Check sheet for the modelled part. Datum: model origin and axes. Units: mm. Face numbers are marked on the shaded views. A direction names the side the tool comes from. Round coordinates to 2 decimals unless told otherwise and drop trailing zeros. Order: outer loops, then holes, each group sorted by start corner. A loop starts at its lowest first (then second) coordinate and runs counter-clockwise, first axis right, second up. Notation, with made-up numbers: (-20, 56.5) -> (37, 56.5) arc R16 cw to (37, 60.5) -> close; hole circle Ø8 at (38, -35.5). An arc over 180 degrees is marked (long way). Answer in a Markdown table with one row per item. Add a question column.
1. Access from +Z, -Z, +X, -X, +Y, -Y to the whole of each face (thin tool, end or side, straight path). Record for the marked faces 1 and 2.
2. Material ranges on L1, parallel to Z at x = -0.5, y = 2.25; L2, parallel to Z at x = 1.25, y = 0; L3, parallel to X at y = 1.25, z = 11, recorded low to high. Write a range as from..to.
3. Depth check by flat-ended pin: P1, Ø1, axis at x = -2, y = -1, coming from the -Z side; P2, Ø1, axis at x = -1.5, z = 5, coming from the -Y side. Enter the tip coordinate at first touch or a pass-through.
4. Sectioned sample at D-D, the plane z = 9.75. Record the boundary of the cut face in (x, y), then the cut area to 3 significant figures.
5. Draft check along Y on the marked faces 3, 4 and 5. Enter one of: +Y half, -Y half, draft (parallel to the pull), parting line (faces both ways), or undercut.
6. Sectioned sample at C-C, the plane z = 1.5. Record the boundary of the cut face in (x, y).
7. Sectioned sample at A-A, the plane y = 0. Record the boundary of the cut face in (x, z).
8. Sectioned sample at B-B, the plane x = 1.25. Record the boundary of the cut face in (y, z).
```python
from build123d import *

# Parameters (mm, degrees)
SKETCH_1_R          = 1.5
EXTRUDE_1_DEPTH     = 6
SKETCH_2_R          = 2
EXTRUDE_2_DEPTH     = 8
SKETCH_3_R          = 3.5
EXTRUDE_3_DEPTH     = 3.5
CUT_EXTRUDE_1_DEPTH = 2


with BuildPart() as part:
    # 草图1 → 凸台-拉伸1 (new body)
    with BuildSketch(Plane.XY):
        Circle(SKETCH_1_R)
    extrude(amount=EXTRUDE_1_DEPTH)

    # 草图2 → 凸台-拉伸2 (add)
    with BuildSketch(Plane.XY.offset(6)):
        Circle(SKETCH_2_R)
    extrude(amount=EXTRUDE_2_DEPTH)

    # 草图3 → 凸台-拉伸3 (add)
    with BuildSketch(Plane.XY.offset(14)):
        Circle(SKETCH_3_R)
    extrude(amount=EXTRUDE_3_DEPTH)

    # 草图4 → 切除-拉伸1 (cut)
    with BuildSketch(Plane.XY.offset(17.5)):
        Polygon((0, 1.905255888), (-1.65, 0.952627944), (-1.65, -0.952627944), (0, -1.905255888), (1.65, -0.952627944), (1.65, 0.952627944), align=None)
    extrude(amount=-CUT_EXTRUDE_1_DEPTH, mode=Mode.SUBTRACT)


solid = part.part
```
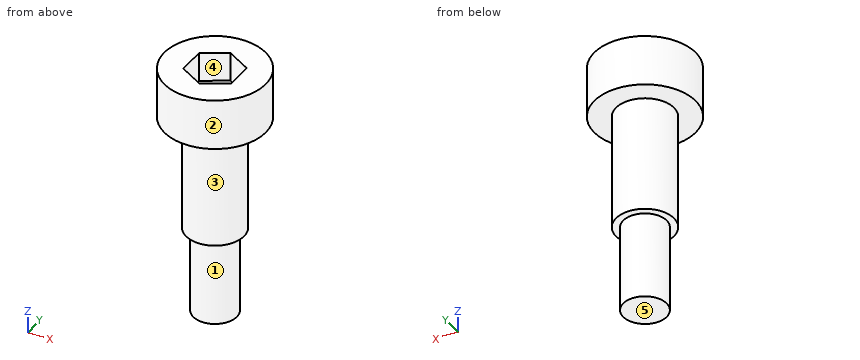
Answer key:
| question | item | result |
|---|---|---|
| 1 | face 1 | -Z |
| 1 | face 2 | +Z, -Z |
| 2 | L1 | z = 14..17.5 |
| 2 | L2 | z = 0..15.5 |
| 2 | L3 | x = -1.56..1.56 |
| 3 | P1 | stops at z = 6 |
| 3 | P2 | stops at y = -1.12 |
| 4 | outline | circle Ø4 at (0, 0) |
| 4 | area | 12.6 mm² |
| 5 | face 3 | parting line |
| 5 | face 4 | undercut |
| 5 | face 5 | draft |
| 6 | outline | circle Ø3 at (0, 0) |
| 7 | outline | (-3.5, 14) -> (-2, 14) -> (-2, 6) -> (-1.5, 6) -> (-1.5, 0) -> (1.5, 0) -> (1.5, 6) -> (2, 6) -> (2, 14) -> (3.5, 14) -> (3.5, 17.5) -> (1.65, 17.5) -> (1.65, 15.5) -> (-1.65, 15.5) -> (-1.65, 17.5) -> (-3.5, 17.5) -> close |
| 8 | outline | (-3.27, 14) -> (-1.56, 14) -> (-1.56, 6) -> (-0.83, 6) -> (-0.83, 0) -> (0.83, 0) -> (0.83, 6) -> (1.56, 6) -> (1.56, 14) -> (3.27, 14) -> (3.27, 17.5) -> (1.18, 17.5) -> (1.18, 15.5) -> (-1.18, 15.5) -> (-1.18, 17.5) -> (-3.27, 17.5) -> close |
